The listing builds one solid part. Answer for the finished solid, in the listing's coordinates (mm). A direction names the side the tool comes from. Give positions to 0.01 mm unless a question says otherwise; leave off trailing zeros. Write each loop counter-clockwise with the first axis right and the second up, starting at its lowest first coordinate (ties: lowest second). Pieces come first, ordered by that corner, then holes. Notation, with made-up numbers: (58.25, 62) -> (79.25, 62) arc R19 ccw to (79.25, 78) -> close; hole circle Ø4 at (8, 23.5). An arc over 180 degrees is marked (long way). Put each result on its own line as item: value. Start each with the question number.
1) A cutting plane is placed at B-B (y = 0). Write down the section's boundary in (x, z).
2) For faces 1 (the cylindrical face through (2.4, -9, -0.4)), 2 (the flat face through (-10, -10.5, 7)), 3 (the flat face through (13, -10.5, 7)), determine the directions among +Z, -Z, +X, -X, +Y, -Y from which every point of the face is accessible in a straight line to the end or side of a thin tool.
3) A cutting plane is placed at C-C (z = 2.75). Write down the section's boundary in (x, y), then the cut area to 3 significant figures.
4) A cutting plane is placed at D-D (x = -8.5). Write down the section's boundary in (y, z).
5) Flat-ended cylindrical pins translate along their axes: pin 1 Ø7 at (x, y) = (-2.5, -5) entering from +Z; pin 2 Ø1.8 at (x, z) = (-10, 5.5) entering from -Y; pin 3 Ø4 at (x, y) = (-10.5, -10.5) entering from -Z. Find the tip coordinate at first contact, or state that the pin passes through.
6) Find the intervals of material crossed by line 1 along Y through (x, z) = (2.5, 4.5); line 2 along X through (y, z) = (-42, 7.75); line 3 along Z through (x, y) = (0, -7.5), in increasing order. Write a range as from..to.
from build123d import *

# Parameters (mm, degrees)
SKETCH_2_R               = 1.65
EXTRUDE_1_DEPTH          = 15
SKETCH_4_W               = 10
SKETCH_4_H               = 21
EXTRUDE_2_DEPTH          = 37.5
CUT_EXTRUDE_1_DEPTH      = 54.011791141
CUT_EXTRUDE_1_DEPTH_BACK = 54.011791141
SKETCH_5_R               = 2
FILLET_1_R               = 3
FILLET_2_R               = 3
FILLET_3_R               = 5


with BuildPart() as part:
    # 草图2 → 凸台-拉伸1 (new body)
    with BuildSketch(Plane.XY):
        Polygon((-13.5, -7.5), (-13.5, 7.5), (13.5, 7.5), (13.5, -7.5), (13.5, -10.5), (-13.5, -10.5), align=None)
        with Locations((7.5, 0)):
            Circle(SKETCH_2_R, mode=Mode.SUBTRACT)
        with Locations((-7.5, 0)):
            Circle(SKETCH_2_R, mode=Mode.SUBTRACT)
    extrude(amount=EXTRUDE_1_DEPTH)

    # 草图4 → 凸台-拉伸2 (add)
    with BuildSketch(Plane.XZ.offset(10.5)):
        with Locations((2.5, 7.5)):
            Rectangle(SKETCH_4_W, SKETCH_4_H)
    extrude(amount=EXTRUDE_2_DEPTH)

    # 草图5 → 切除-拉伸1 (cut, two sides: drawn at the far end of the back side and taken through both)
    with BuildSketch(Plane(origin=(0, 0, 0), x_dir=(-1, 0, 0), z_dir=(0, 0, -1)).offset(-CUT_EXTRUDE_1_DEPTH_BACK)):
        with Locations((-2.5, -42)):
            Circle(SKETCH_5_R)
    extrude(amount=CUT_EXTRUDE_1_DEPTH + CUT_EXTRUDE_1_DEPTH_BACK, mode=Mode.SUBTRACT)

    # 圆角1
    fillet_1_edges = [part.edges().sort_by_distance(p)[0] for p in [
        (4.5, -42, 18),
        (2.5, -10.5, 0),
        (2.5, -10.5, 15),
        (4.5, -42, -3),
    ]]
    fillet(fillet_1_edges, radius=FILLET_1_R - 0.0001)  # a hair under: the kernel refuses the full size

    # 圆角2
    fillet_2_edges = [part.edges().sort_by_distance(p)[0] for p in [
        (2.5, -10.5, -3),
        (2.5, -10.5, 18),
    ]]
    fillet(fillet_2_edges, radius=FILLET_2_R)

    # 圆角3
    fillet_3_edges = [part.edges().sort_by_distance(p)[0] for p in [
        (7.5, -10.5, 7.5),
        (-2.5, -10.5, 7.5),
    ]]
    fillet(fillet_3_edges, radius=FILLET_3_R)


solid = part.part
Reply:
1. outline: (-13.5, 0) -> (-9.15, 0) -> (-9.15, 15) -> (-13.5, 15) -> close; (-5.85, 0) -> (5.85, 0) -> (5.85, 15) -> (-5.85, 15) -> close; (9.15, 0) -> (13.5, 0) -> (13.5, 15) -> (9.15, 15) -> close
2. face 1: -Z, +X, -X, +Y
2. face 2: +Z, -Z, -X, -Y
2. face 3: +Z, -Z, +X, -Y
3. outline: (-13.5, -10.5) -> (-7.5, -10.5) arc R5 cw to (-2.5, -15.5) -> (-2.5, -48) -> (7.5, -48) -> (7.5, -15.5) arc R5 cw to (12.5, -10.5) -> (13.5, -10.5) -> (13.5, 7.5) -> (-13.5, 7.5) -> close; hole circle Ø3.3 at (-7.5, 0); hole circle Ø4 at (2.5, -42); hole circle Ø3.3 at (7.5, 0)
3. area: 842 mm2
4. outline: (-10.5, 0) -> (-1.31, 0) -> (-1.31, 15) -> (-10.5, 15) -> close; (1.31, 0) -> (7.5, 0) -> (7.5, 15) -> (1.31, 15) -> close
5. pin 1: stops at z = 15.17
5. pin 2: stops at y = -10.5
5. pin 3: stops at z = 0
6. line 1: y = -48..-44, -40..7.5
6. line 2: x = -2.5..0.5, 4.5..7.5
6. line 3: z = 0..15
